from build123d import *

# Parameters (mm, degrees)
SKETCH1_W                 = 56.4
SKETCH1_H                 = 26
BOSS_EXTRUDE1_DEPTH       = 5
F_2_0MM_DOWEL_HOLE1_D     = 2
F_2_0MM_DOWEL_HOLE1_DEPTH = 7
F_2_0MM_DOWEL_HOLE1_TIP   = 0.600860619
F_2_0MM_DOWEL_HOLE2_D     = 2
F_2_0MM_DOWEL_HOLE2_DEPTH = 7
F_2_0MM_DOWEL_HOLE2_TIP   = 0.600860619
F_2_5MM_DOWEL_HOLE1_D     = 2.5
F_2_5MM_DOWEL_HOLE1_DEPTH = 8
F_2_5MM_DOWEL_HOLE1_TIP   = 0.751075774


with BuildPart() as part:
    # Sketch1 → Boss-Extrude1 (new body)
    with BuildSketch(Plane(origin=(0, 0, 0), x_dir=(1, 0, 0), z_dir=(0, 1, 0))):
        with Locations((28.2, 13)):
            Rectangle(SKETCH1_W, SKETCH1_H)
    extrude(amount=BOSS_EXTRUDE1_DEPTH)

    # Ø2.0mm Dowel Hole1
    with Locations(Plane(origin=(56.4, 0, 0), x_dir=(0, 0, -1), z_dir=(1, 0, 0))):
        with Locations((6.5, 2.5), (13, 2.5), (19.5, 2.5)):
            Hole(F_2_0MM_DOWEL_HOLE1_D / 2, depth=F_2_0MM_DOWEL_HOLE1_DEPTH)
            with Locations((0, 0, -(F_2_0MM_DOWEL_HOLE1_DEPTH + F_2_0MM_DOWEL_HOLE1_TIP / 2))):  # 118° drill point
                Cone(0, F_2_0MM_DOWEL_HOLE1_D / 2, F_2_0MM_DOWEL_HOLE1_TIP, mode=Mode.SUBTRACT)

    # Ø2.0mm Dowel Hole2
    with Locations(Plane.ZY):
        with Locations((-19.5, 2.5), (-13, 2.5), (-6.5, 2.5)):
            Hole(F_2_0MM_DOWEL_HOLE2_D / 2, depth=F_2_0MM_DOWEL_HOLE2_DEPTH)
            with Locations((0, 0, -(F_2_0MM_DOWEL_HOLE2_DEPTH + F_2_0MM_DOWEL_HOLE2_TIP / 2))):  # 118° drill point
                Cone(0, F_2_0MM_DOWEL_HOLE2_D / 2, F_2_0MM_DOWEL_HOLE2_TIP, mode=Mode.SUBTRACT)

    # Ø2.5mm Dowel Hole1
    with Locations(Plane(origin=(21.27179677, 5, -9), x_dir=(0, 0, 1), z_dir=(0, 1, 0))):
        with Locations((0, 0), (-12, 6.92820323), (0, 13.85640646)):
            Hole(F_2_5MM_DOWEL_HOLE1_D / 2, depth=F_2_5MM_DOWEL_HOLE1_DEPTH)
            with Locations((0, 0, -(F_2_5MM_DOWEL_HOLE1_DEPTH + F_2_5MM_DOWEL_HOLE1_TIP / 2))):  # 118° drill point
                Cone(0, F_2_5MM_DOWEL_HOLE1_D / 2, F_2_5MM_DOWEL_HOLE1_TIP, mode=Mode.SUBTRACT)


solid = part.part
Read the model definition and answer for the solid it produces. Units are mm, in the model's axes. A direction names the side the tool comes from. Coordinates: 2 decimals unless noted, no trailing zeros. Loops run counter-clockwise (first coordinate to the right, second up) from the corner with the lowest first, then second, coordinate; pieces in that order, holes last. Notation, with made-up numbers: (-33, 6.25) - (-22, 6.25) arc R19 cw to (-22, 21.25) - close; hole circle Ø8 at (49, -26.75). An arc over 180 degrees is marked (long way). Answer in a Markdown table with one row per item.
Q1. For faces 1 (the cylindrical face through (35.973, 2.465, -8.079)), 2 (the cylindrical face through (52.9, 2.5, -7.5)), 3 (the cylindrical face through (3.5, 2.5, -5.5)), determine the directions among +Z, -Z, +X, -X, +Y, -Y from which every point of the face is accessible in a straight line to the end or side of a thin tool.
Here are the results:
| item | result |
|---|---|
| face 1 | +Y, -Y |
| face 2 | +X |
| face 3 | -X |
Q2. Given P1, Ø1.2, axis at y = 2.5, z = -6.5, coming from the +X side, flat-ended and moving along its own axis, determine where the tip first touches the part or whether it passes through.
Here are the results:
| item | result |
|---|---|
| P1 | stops at x = 49.16 |
Q3. Straight lines are drawn through the part: line 1 along X through (y, z) = (1.9, -9); line 2 along Z through (x, y) = (4, 2.5); line 3 along Y through (x, z) = (52.75, -19.5). For each, find the intervals that lie inside material, in ascending order. Write a range as [from, to].
Here are the results:
| item | result |
|---|---|
| line 1 | x = [0, 20.02], [22.52, 33.88], [36.38, 56.4] |
| line 2 | z = [-26, -20.5], [-18.5, -14], [-12, -7.5], [-5.5, 0] |
| line 3 | y = [0, 1.5], [3.5, 5] |
Q4. The mould has two halves that part along Z. Classify faces 4 (the flat face through (28, 2, 0)), 5 (the cylindrical face through (52.851, 2.8, -12.046)), 6 (the flat face through (28, 0, -13)), 7 (the conical face through (48.9, 2.51, -6.33)): pulls with the +Z half, pulls with the -Z half, needs draft (parallel to the pull), parting line crosses it, or undercut.
Here are the results:
| item | result |
|---|---|
| face 4 | pulls with the +Z half |
| face 5 | undercut |
| face 6 | needs draft |
| face 7 | undercut |
Q5. Find section C-C on x = 27.5. Write down the section's boundary in (y, z).
Here are the results:
| item | result |
|---|---|
| outline | (0, -26) - (5, -26) - (5, -22.04) - (0, -22.04) - close; (0, -19.96) - (5, -19.96) - (5, 0) - (0, 0) - close |
Q6. Find section B-B on z = -21. Write down the section's boundary in (x, y), plus the area to 4 significant figures.
Here are the results:
| item | result |
|---|---|
| outline | (0, 0) - (26.95, 0) - (26.95, 5) - (0, 5) - close; (29.45, 0) - (56.4, 0) - (56.4, 5) - (29.45, 5) - close |
| area | 269.5 mm^2 |
Q7. Find section A-A on z = -9. Write down the section's boundary in (x, y), plus the area to 3 significant figures.
Here are the results:
| item | result |
|---|---|
| outline | (0, 0) - (20.02, 0) - (20.02, 5) - (0, 5) - close; (22.52, 0) - (33.88, 0) - (33.88, 5) - (22.52, 5) - close; (36.38, 0) - (56.4, 0) - (56.4, 5) - (36.38, 5) - close |
| area | 257 mm^2 |
